from build123d import *

# Parameters (mm, degrees)
SKETCH_1_R      = 33.5
SKETCH_1_R_2    = 12.625
SKETCH_1_R_3    = 2
SKETCH_1_R_4    = 1.4
EXTRUDE_1_DEPTH = 1


with BuildPart() as part:
    # 草图1 → 凸台-拉伸1 (new body)
    with BuildSketch(Plane.XY):
        Circle(SKETCH_1_R)
        Circle(SKETCH_1_R_2, mode=Mode.SUBTRACT)
        with Locations((0, -28)):
            Circle(SKETCH_1_R_3, mode=Mode.SUBTRACT)
        with Locations((-26.629582456, -8.652475842)):
            Circle(SKETCH_1_R_3, mode=Mode.SUBTRACT)
        with Locations((-16.457987064, 22.652475842)):
            Circle(SKETCH_1_R_3, mode=Mode.SUBTRACT)
        with Locations((16.457987064, 22.652475842)):
            Circle(SKETCH_1_R_3, mode=Mode.SUBTRACT)
        with Locations((26.629582456, -8.652475842)):
            Circle(SKETCH_1_R_3, mode=Mode.SUBTRACT)
        with Locations((-11.755705046, -16.180339887)):
            Circle(SKETCH_1_R_4, mode=Mode.SUBTRACT)
        with Locations((-19.021130326, 6.180339887)):
            Circle(SKETCH_1_R_4, mode=Mode.SUBTRACT)
        with Locations((0, 20)):
            Circle(SKETCH_1_R_4, mode=Mode.SUBTRACT)
        with Locations((19.021130326, 6.180339887)):
            Circle(SKETCH_1_R_4, mode=Mode.SUBTRACT)
        with Locations((11.755705046, -16.180339887)):
            Circle(SKETCH_1_R_4, mode=Mode.SUBTRACT)
    extrude(amount=EXTRUDE_1_DEPTH)


solid = part.part
For this review, take the finished solid that the model builds, in its own axes (mm). Give positions to 0.01 mm unless a question says otherwise; leave off trailing zeros. Loops run counter-clockwise (first coordinate to the right, second up) from the corner with the lowest first, then second, coordinate; pieces in that order, holes last. Notation, with made-up numbers: M 12.5,86 L 21.5,86 A19 ccw 21.5,118 Z; hole C 85,-11 d5. An arc over 180 degrees is marked long. Answer as a JSON object with one key per item and string values. Group by question number.
Q1. Add section A-A on y = 0. Give the boundary of the cut face in (x, z) (3 decimals), and give its area (4 significant figures).
Q2. Insertion check: P1, Ø3.5, axis at x = -16.46, y = 22.65, coming from the +Z side. The pin has a flat end and moves straight along its axis. Give the tip position at first contact, or say it passes through.
Q3. For probe 1 along Y at (x, z) = (0, 0.6) (3 decimals); probe 2 along X at (y, z) = (-15, 0.85); probe 3 along Y at (x, z) = (-4, 0.6), list the stretches that pass through material, from the lowest coordinate up. Write a range as [from, to].
Q4. Add section D-D on y = -28. Give the boundary of the cut face in (x, z).
Q5. Mouldability with a two-part tool opening along X and no side actions: class faces 1 (the flat face through (14, 0, 0)), 2 (the cylindrical face through (-13.154, -16.119, 0.493)), 3 (the cylindrical face through (-7.262, -32.703, 0.493)) as +X half, -X half, draft (parallel to the pull), parting line (faces both ways), or undercut.
Q6. Add section B-B on x = 0. Give the boundary of the cut face in (y, z) (3 decimals), and give its area (4 significant figures).
Q7. Add section C-C on z = 0.35. Give the number of separate pieces and of enclosed holes in the cut face, and give its area (3 significant figures).
Checked values:
{
 "1": {"outline": "M -33.5,0 L -12.625,0 L -12.625,1 L -33.5,1 Z; M 12.625,0 L 33.5,0 L 33.5,1 L 12.625,1 Z", "area": "41.75 mm²"},
 "2": {"P1": "through"},
 "3": {"probe 1": "[-33.5, -30], [-26, -12.625], [12.625, 18.6], [21.4, 33.5]", "probe 2": "[-29.95, -12.51], [-11, 11], [12.51, 29.95]", "probe 3": "[-33.26, -11.97], [11.97, 33.26]"},
 "4": {"outline": "M -18.39,0 L -2,0 L -2,1 L -18.39,1 Z; M 2,0 L 18.39,0 L 18.39,1 L 2,1 Z"},
 "5": {"face 1": "draft", "face 2": "undercut", "face 3": "parting line"},
 "6": {"outline": "M -33.5,0 L -30,0 L -30,1 L -33.5,1 Z; M -26,0 L -12.625,0 L -12.625,1 L -26,1 Z; M 12.625,0 L 18.6,0 L 18.6,1 L 12.625,1 Z; M 21.4,0 L 33.5,0 L 33.5,1 L 21.4,1 Z", "area": "34.95 mm²"},
 "7": {"separate pieces": "1", "enclosed holes": "11", "area": "2,930 mm²"}
}
